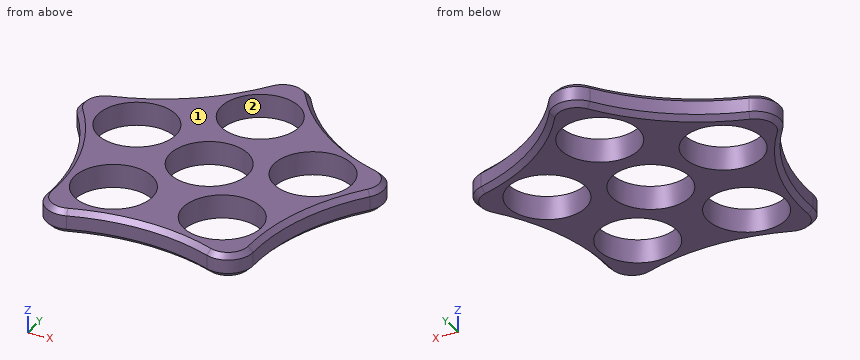
```python
from build123d import *

# Parameters (mm, degrees)
F0_R     = 7.9375
F1_DEPTH = 4.826
F2_R     = 5.08
F3_SIZE  = 1.016


with BuildPart() as f1:
    # F0 (on Top) → F1 (new body)
    with BuildSketch(Plane.XY):
        with BuildLine():
            ThreePointArc((-36.2352532708, 11.7735474857), (-23.2757268131, -7.5627420857), (-22.3946181123, -30.8235474857))
            ThreePointArc((-22.3946181123, -30.8235474857), (0, -24.4735474857), (22.3946181123, -30.8235474857))
            ThreePointArc((22.3946181123, -30.8235474857), (23.2757268131, -7.5627420857), (36.2352532708, 11.7735474857))
            ThreePointArc((36.2352532708, 11.7735474857), (14.3851902834, 19.7995158286), (0, 38.1))
            ThreePointArc((0, 38.1), (-14.3851902834, 19.7995158286), (-36.2352532708, 11.7735474857))
        make_face()
        with Locations((-11.1973090562, -15.4117737428)):
            Circle(F0_R, mode=Mode.SUBTRACT)
        Circle(F0_R, mode=Mode.SUBTRACT)
        with Locations((11.1973090562, -15.4117737428)):
            Circle(F0_R, mode=Mode.SUBTRACT)
        with Locations((-18.1176266354, 5.8867737428)):
            Circle(F0_R, mode=Mode.SUBTRACT)
        with Locations((0, 19.05)):
            Circle(F0_R, mode=Mode.SUBTRACT)
        with Locations((18.1176266354, 5.8867737428)):
            Circle(F0_R, mode=Mode.SUBTRACT)
    extrude(amount=F1_DEPTH)

    # F2
    f2_edges = [f1.edges().sort_by_distance(p)[0] for p in [
        (0, 38.1, 2.413),
        (36.235253, 11.773547, 2.413),
        (22.394618, -30.823547, 2.413),
        (-22.394618, -30.823547, 2.413),
        (-36.235253, 11.773547, 2.413),
    ]]
    fillet(f2_edges, radius=F2_R)

    # F3
    f3_edges = [f1.edges().sort_by_distance(p)[0] for p in [
        (-30.929782, 10.049695, 0),
        (-23.275727, -7.562742, 4.826),
    ]]
    chamfer(f3_edges, length=F3_SIZE)


solid = f1.part
```
The model under review builds one solid part; all positions refer to its coordinate system, in mm. Face numbers are marked on the shaded views. Give positions to 0.01 mm unless a question says otherwise; leave off trailing zeros. Answer in a Markdown table with one row per item.
1) Mouldability with a two-part tool opening along Y and no side actions: class the marked faces 1 and 2 as +Y half, -Y half, draft (parallel to the pull), parting line (faces both ways), or undercut.
Worked answers:
| item | result |
|---|---|
| face 1 | draft |
| face 2 | undercut |
2) Clearance check with flat-ended pins moving along their axes: P1, Ø2, axis at y = -0.5, z = 1, coming from the -X side; P2, Ø1, axis at x = -12.5, z = 3, coming from the +Y side; P3, Ø9.5, axis at x = 0, y = 0, coming from the +Z side; P4, Ø12, axis at x = 21.5, y = 1.5, coming from the -Z side. State where each tip first meets the part, or that it passes through.
Worked answers:
| item | result |
|---|---|
| P1 | x = -26.85 |
| P2 | y = 21.67 |
| P3 | through |
| P4 | z = 0 |
3) For L1, parallel to Y at x = 0, z = 2.65; L2, parallel to X at y = -15.5, z = 2.75; L3, parallel to X at y = -14.5, z = 4.55, list the stretches that pass through material, from the lowest coordinate up. Write a range as [from, to].
Worked answers:
| item | result |
|---|---|
| L1 | [-24.47, -7.94], [7.94, 11.11], [26.99, 32.52] |
| L2 | [-21.51, -19.13], [-3.26, 3.26], [19.13, 21.51] |
| L3 | [-20.9, -19.08], [-3.31, 3.31], [19.08, 20.9] |
4) Add section A-A on x = 0. Count the separate pieces of the cut face and the enclosed holes in it, plus the area to 3 significant figures.
Worked answers:
| item | result |
|---|---|
| separate pieces | 3 |
| enclosed holes | 0 |
| area | 120 mm² |
